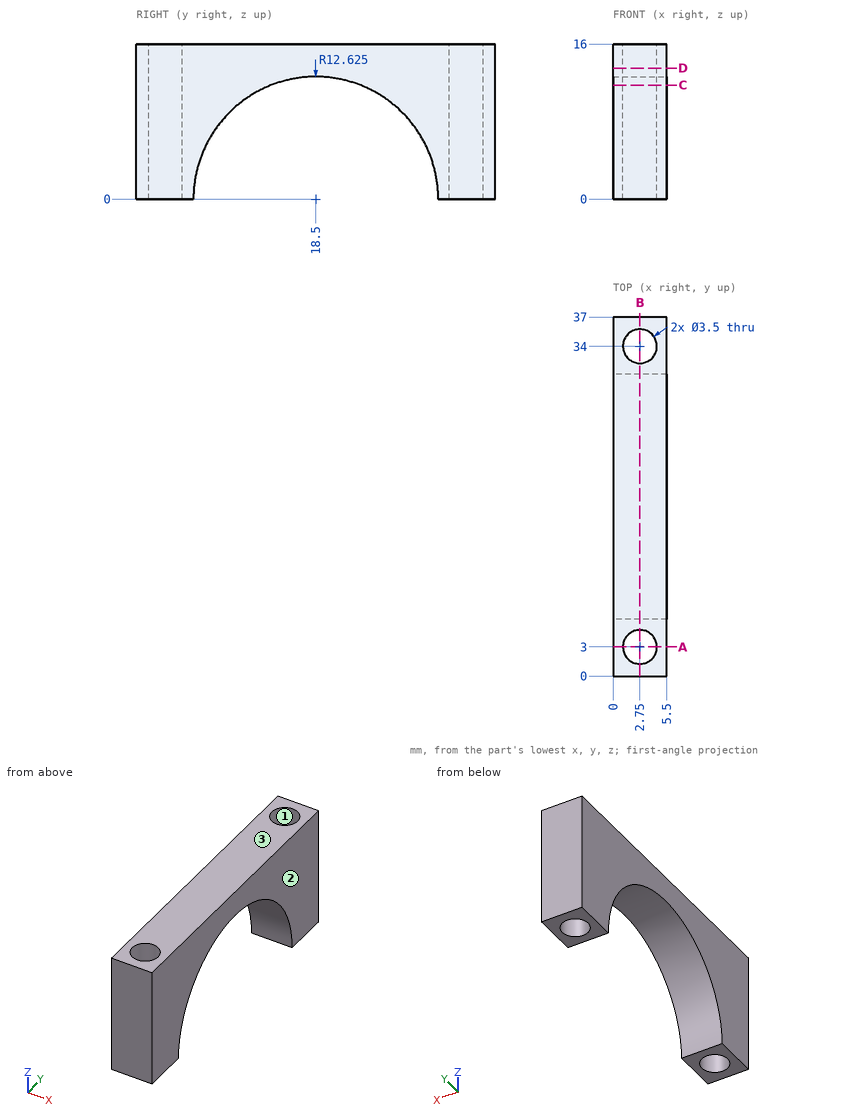
Source: three-view drawing plus pictorial views. Frame: mm from the lowest corner of the part. Give positions to 0.01 mm unless a question says otherwise; leave off trailing zeros. Order: outer loops, then holes, each group sorted by start corner. A loop starts at its lowest first (then second) coordinate and runs counter-clockwise, first axis right, second up. Notation, with made-up numbers: (47.5, 21) - (88.5, 21) arc R27 ccw to (88.5, 39) - close; hole circle Ø4 at (-15.75, 25.25). An arc over 180 degrees is marked (long way). Put each result on its own line as item: value.
Item 1: Contact query for flat-ended pins moving along their axis: pin 1 (6 mm diameter, centred on y = 25.5, z = 5.5, fed in from -X); pin 2 (1 mm diameter, centred on x = 2.5, y = 10, fed in from -Z). Output: stop coordinate, or through.
Found:
pin 1: passes through
pin 2: stops at z = 8.85
Item 2: Section query A-A, the plane y = 3. Return loops of the section in (x, z), then the cut area to 3 significant figures.
Found:
outline: (0, 0) - (1, 0) - (1, 16) - (0, 16) - close; (4.5, 0) - (5.5, 0) - (5.5, 16) - (4.5, 16) - close
area: 32.0 mm^2
Item 3: Section query C-C, the plane z = 11.75. Return loops of the section in (x, y), then the cut area to 3 significant figures.
Found:
outline: (0, 0) - (5.5, 0) - (5.5, 13.88) - (0, 13.88) - close; (0, 23.12) - (5.5, 23.12) - (5.5, 37) - (0, 37) - close; hole circle Ø3.5 at (2.75, 3); hole circle Ø3.5 at (2.75, 34)
area: 133 mm^2
Item 4: Section query B-B, the plane x = 2.75. Return loops of the section in (y, z) (3 decimals).
Found:
outline: (0, 0) - (1.25, 0) - (1.25, 16) - (0, 16) - close; (4.75, 0) - (5.875, 0) arc R12.625 cw to (31.125, 0) - (32.25, 0) - (32.25, 16) - (4.75, 16) - close; (35.75, 0) - (37, 0) - (37, 16) - (35.75, 16) - close
Item 5: Ray query, L1, parallel to Y at x = 2.75, z = 9.75; L2, parallel to Y at x = 3.4, z = 4; L3, parallel to X at y = 3, z = 8.5. Return the intervals inside material, ascending. Write a range as from..to.
Found:
L1: y = 0..1.25, 4.75..10.48, 26.52..32.25, 35.75..37
L2: y = 0..1.38, 4.62..6.53, 30.47..32.38, 35.62..37
L3: x = 0..1, 4.5..5.5
Item 6: Draft query along X for the marked faces 1, 2 and 3. Return one class per face: +X half, -X half, draft (parallel to the pull), parting line (faces both ways), or undercut.
Found:
face 1: undercut
face 2: +X half
face 3: draft
Item 7: Section query D-D, the plane z = 13.5. Return loops of the section in (x, y).
Found:
outline: (0, 0) - (5.5, 0) - (5.5, 37) - (0, 37) - close; hole circle Ø3.5 at (2.75, 3); hole circle Ø3.5 at (2.75, 34)
